Can you work these out from the drawing? Everything is in mm from the part's minimum corner. A direction names the side the tool comes from. Coordinates: 2 decimals unless noted, no trailing zeros. Order: outer loops, then holes, each group sorted by start corner. A loop starts at its lowest first (then second) coordinate and runs counter-clockwise, first axis right, second up. Notation, with made-up numbers: M -13.75,-32.75 L 17.25,-32.75 A17 ccw 17.25,-24.75 Z; hole C 78.5,-7.5 d4. An arc over 180 degrees is marked long. One line per question, with ' | ' between items. Start each with the question number.
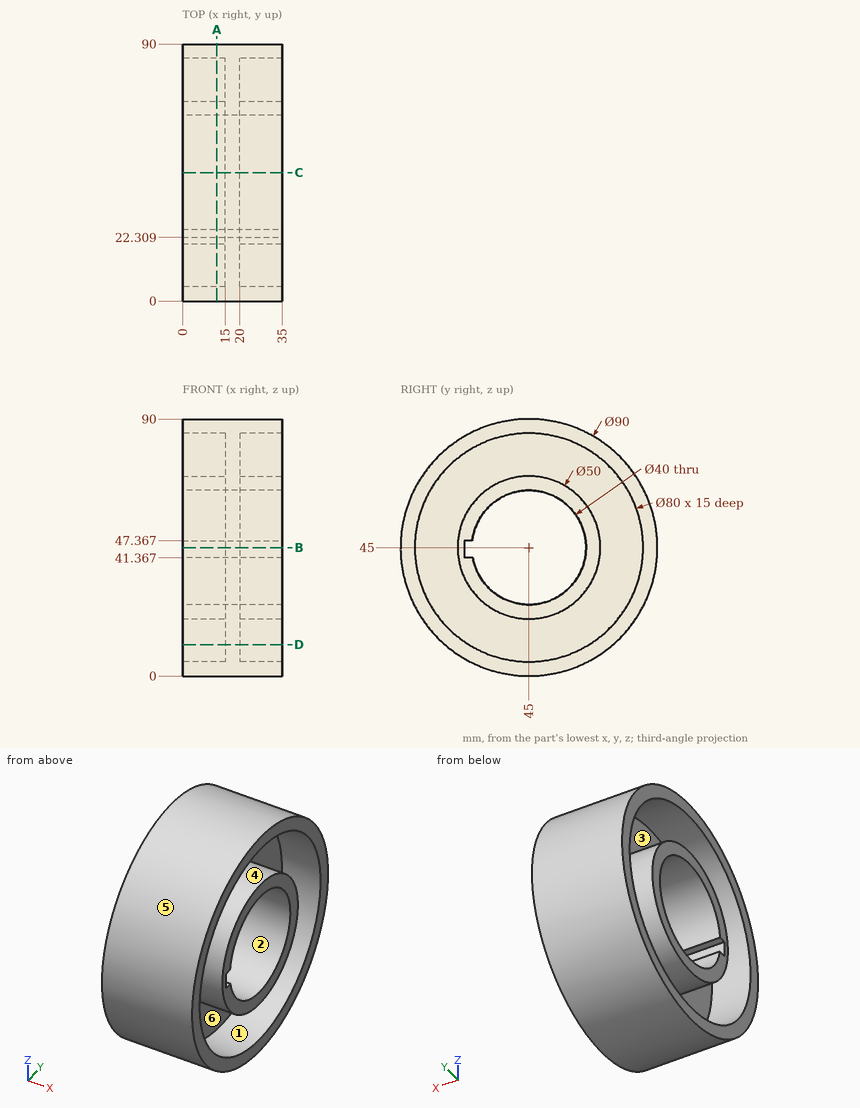
(1) We'd pull the mould along Y, two halves only. Please class the marked faces 4, 5 and 6: +Y half, -Y half, draft (parallel to the pull), parting line (faces both ways), or undercut.
(2) Imagine slicing it at D-D, the plane z = 11. Write out the boundary of the cut face in (x, y).
(3) If I drill on line 1 along Y through (x, z) = (5.25, 45); line 2 along Z through (x, y) = (29, 46) (1 decimal); line 3 along Y through (x, z) = (23.5, 30) (1 decimal), over which ranges is the centre line in solid material (lowest first)? Write a range as from..to.
(4) Imagine slicing it at C-C, the plane y = 45. Write out the boundary of the cut face in (x, z).
(5) For P1, Ø1.4, axis at x = 11.5, y = 23.5, coming from the -Z side (1 decimal); P2, Ø3, axis at x = 14.5, y = 12, coming from the +Z side; P3, Ø3, axis at y = 77, z = 53, coming from the -X side, each with a flat end and sliding along its axis, tell me the tip position at first contact or that it passes through.
(6) Imagine slicing it at B-B, the plane z = 45. Write out the boundary of the cut face in (x, y).
(7) On a 3-axis mill with a long thin cutter (end or side, diameter ignored), from which of +Z, -Z, +X, -X, +Y, -Y can I reach the whole of each face in a straight line? I mean the marked faces 1, 2 and 3. Say none if no direction works.
(8) Imagine slicing it at A-A, the plane x = 12. Write out the boundary of the cut face in (y, z).
Answers:
1) face 4: undercut | face 5: parting line | face 6: undercut
2) outline: M 0,15.52 L 35,15.52 L 35,23.93 L 20,23.93 L 20,66.07 L 35,66.07 L 35,74.48 L 0,74.48 L 0,66.07 L 15,66.07 L 15,23.93 L 0,23.93 Z
3) line 1: 0..5, 20..22.31, 65..70, 85..90 | line 2: 0..5, 20..25, 65..70, 85..90 | line 3: 2.6..7.9, 25..31.8, 58.2..65, 82.1..87.4
4) outline: M 0,0 L 35,0 L 35,5 L 20,5 L 20,20 L 35,20 L 35,25 L 0,25 L 0,20 L 15,20 L 15,5 L 0,5 Z; M 0,65 L 35,65 L 35,70 L 20,70 L 20,85 L 35,85 L 35,90 L 0,90 L 0,85 L 15,85 L 15,70 L 0,70 Z
5) P1: z = 5.1 | P2: z = 77.14 | P3: x = 15
6) outline: M 0,0 L 35,0 L 35,5 L 20,5 L 20,20 L 35,20 L 35,22.31 L 0,22.31 L 0,20 L 15,20 L 15,5 L 0,5 Z; M 0,65 L 35,65 L 35,70 L 20,70 L 20,85 L 35,85 L 35,90 L 0,90 L 0,85 L 15,85 L 15,70 L 0,70 Z
7) face 1: +X | face 2: +X, -X | face 3: -X
8) outline: C 45,45 d90; C 45,45 d50; hole C 45,45 d80; hole M 22.31,41.37 L 25.33,41.37 A20 ccw long 25.14,47.37 L 22.31,47.37 Z
